Check sheet for the modelled part. Datum: model origin and axes. Units: mm. A direction names the side the tool comes from. Give positions to 0.01 mm unless a question says otherwise; leave off trailing zeros. Loops run counter-clockwise (first coordinate to the right, second up) from the corner with the lowest first, then second, coordinate; pieces in that order, holes last.
```python
from build123d import *

# Parameters (mm, degrees)
EXTRUDE_1_DEPTH          = 245
CUT_EXTRUDE_2_DEPTH      = 249.646335183
CUT_EXTRUDE_2_DEPTH_BACK = 249.646335183
SKETCH_3_R               = 2


with BuildPart() as part:
    # 草图1 → 凸台-拉伸1 (new, symmetric)
    with BuildSketch(Plane(origin=(0, 0, 0), x_dir=(1, 0, 0), z_dir=(0, 1, 0))):
        with BuildLine():
            Line((4, 0), (26, 0))
            ThreePointArc((26, 0), (28.828427125, 1.171572875), (30, 4))
            Line((30, 4), (30, 26))
            ThreePointArc((30, 26), (28.828427125, 28.828427125), (26, 30))
            Line((26, 30), (4, 30))
            ThreePointArc((4, 30), (1.171572875, 28.828427125), (0, 26))
            Line((0, 26), (0, 4))
            ThreePointArc((0, 4), (1.171572875, 1.171572875), (4, 0))
        make_face()
        with BuildLine():
            Line((4, 2), (26, 2))
            ThreePointArc((26, 2), (27.414213562, 2.585786438), (28, 4))
            Line((28, 4), (28, 26))
            ThreePointArc((28, 26), (27.414213562, 27.414213562), (26, 28))
            Line((26, 28), (4, 28))
            ThreePointArc((4, 28), (2.585786438, 27.414213562), (2, 26))
            Line((2, 26), (2, 4))
            ThreePointArc((2, 4), (2.585786438, 2.585786438), (4, 2))
        make_face(mode=Mode.SUBTRACT)
    extrude(amount=EXTRUDE_1_DEPTH, both=True)

    # 草图3 → 切除-拉伸2 (cut, two sides: drawn at the far end of the back side and taken through both)
    with BuildSketch(Plane(origin=(0, 0, 0), x_dir=(0, 0, -1), z_dir=(1, 0, 0)).offset(-CUT_EXTRUDE_2_DEPTH_BACK)):
        with Locations(Location((15, -149.5, 0), (0, 0, 180))):
            Circle(SKETCH_3_R)
        with Locations(Location((15, -139.5, 0), (0, 0, 180))):
            Circle(SKETCH_3_R)
        with Locations(Location((15, 139.5, 0), (0, 0, 180))):
            Circle(SKETCH_3_R)
        with Locations(Location((15, 149.5, 0), (0, 0, 180))):
            Circle(SKETCH_3_R)
        with Locations(Location((15, 125, 0), (0, 0, 180))):
            Circle(SKETCH_3_R)
        with Locations(Location((15, 45, 0), (0, 0, 180))):
            Circle(SKETCH_3_R)
        with Locations(Location((15, -45, 0), (0, 0, 180))):
            Circle(SKETCH_3_R)
        with Locations(Location((15, -125, 0), (0, 0, 180))):
            Circle(SKETCH_3_R)
    extrude(amount=CUT_EXTRUDE_2_DEPTH + CUT_EXTRUDE_2_DEPTH_BACK, mode=Mode.SUBTRACT)


solid = part.part
```
(1) Material ranges on line 1 (X direction, y = -170, z = -26.5); line 2 (X direction, y = -191, z = -7); line 3 (Z direction, x = 18, y = 106), recorded low to high.
(2) Release check for a two-part mould opening along X. For faces 3 (the face through (30, 3, -15)), 4 (the face through (15, 3, -28)), 5 (the face through (1, 245, -15)) record: pulls with the +X half, pulls with the -X half, needs draft (parallel to the pull), parting line crosses it, or undercut.
(3) Section check B-B on x = 13. Record the boundary of the cut face in (y, z), plus the area to 3 significant figures.
(4) Section check A-A on y = 195.5. Record the boundary of the cut face in (x, z), plus the area to 3 significant figures.
(5) Access from +Z, -Z, +X, -X, +Y, -Y to the whole of each face (thin tool, end or side, straight path). Record for faces 1 (the face through (15, 3, -30)), 2 (the face through (28, 3, -15)).
(6) Gauge pin test, flat end, axial feed: pin 1 Ø3.5 at (y, z) = (-149.5, -15) entering from -X. Record the tip position at first contact, or that the pin passes through.
Computed values:
1. line 1: x = 0.03 to 2.06, 27.94 to 29.97
1. line 2: x = 0 to 2, 28 to 30
1. line 3: z = -30 to -28, -2 to 0
2. face 3: pulls with the +X half
2. face 4: undercut
2. face 5: needs draft
3. outline: (-245, -30) - (245, -30) - (245, -28) - (-245, -28) - close; (-245, -2) - (245, -2) - (245, 0) - (-245, 0) - close
3. area: 1,960 mm2
4. outline: (0, -26) arc R4 ccw to (4, -30) - (26, -30) arc R4 ccw to (30, -26) - (30, -4) arc R4 ccw to (26, 0) - (4, 0) arc R4 ccw to (0, -4) - close; hole (2, -26) arc R2 ccw to (4, -28) - (26, -28) arc R2 ccw to (28, -26) - (28, -4) arc R2 ccw to (26, -2) - (4, -2) arc R2 ccw to (2, -4) - close
4. area: 214 mm2
5. face 1: -Z, +X, -X, +Y, -Y
5. face 2: +Y, -Y
6. pin 1: passes through
